```python
from build123d import *

# Parameters (mm, degrees)
SKETCH1_W             = 32
SKETCH1_H             = 48
BOSS_EXTRUDE1_DEPTH   = 26
SHELL1_T              = -2
SKETCH2_W             = 26.2
SKETCH2_H             = 24
CUT_EXTRUDE1_DEPTH    = 20
CHAMFER1_SIZE         = 2.5
CHAMFER1_SIZE2        = 2.979383981
CHAMFER1_PART_2_SIZE  = 2.5
CHAMFER1_PART_2_SIZE2 = 2.979383981
CHAMFER3_SIZE         = 2.5
SKETCH5_W             = 27
SKETCH5_H             = 2.432389293
BOSS_EXTRUDE3_DEPTH   = 10
CHAMFER4_SIZE         = 5
SKETCH6_R             = 8.805
CUT_EXTRUDE3_DEPTH    = 10


with BuildPart() as part:
    # Sketch1 → Boss-Extrude1 (new body)
    with BuildSketch(Plane(origin=(0, 0, 0), x_dir=(1, 0, 0), z_dir=(0, 1, 0))):
        Rectangle(SKETCH1_W, SKETCH1_H)
    extrude(amount=BOSS_EXTRUDE1_DEPTH)

    # Shell1
    shell1_openings = [part.faces().sort_by_distance(p)[0] for p in [
        (0, 26, 0),
    ]]
    offset(amount=SHELL1_T, openings=shell1_openings, kind=Kind.INTERSECTION)

    # Sketch2 → Cut-Extrude1 (cut)
    with BuildSketch(Plane(origin=(0, 0, -24), x_dir=(-1, 0, 0), z_dir=(0, 0, -1))):
        with Locations((0, 14)):
            Rectangle(SKETCH2_W, SKETCH2_H)
    extrude(amount=-CUT_EXTRUDE1_DEPTH, mode=Mode.SUBTRACT)

    # Chamfer1
    chamfer1_edges = [part.edges().sort_by_distance(p)[0] for p in [
        (16, 13, 24),
    ]]
    chamfer1_side = [part.faces().sort_by_distance(p)[0] for p in [
        (0, 13, 24),
    ]]
    chamfer(chamfer1_edges, length=CHAMFER1_SIZE, length2=CHAMFER1_SIZE2, reference=chamfer1_side[0])

    # Chamfer1 part 2
    chamfer1_part_2_edges = [part.edges().sort_by_distance(p)[0] for p in [
        (-16, 13, 24),
    ]]
    chamfer1_part_2_side = [part.faces().sort_by_distance(p)[0] for p in [
        (-16, 13, 0),
    ]]
    chamfer(chamfer1_part_2_edges, length=CHAMFER1_PART_2_SIZE, length2=CHAMFER1_PART_2_SIZE2, reference=chamfer1_part_2_side[0])

    # Chamfer3
    chamfer3_edges = [part.edges().sort_by_distance(p)[0] for p in [
        (-16, 13, -24),
        (16, 13, -24),
    ]]
    chamfer(chamfer3_edges, length=CHAMFER3_SIZE)

    # Sketch5 → Boss-Extrude3 (add)
    with BuildSketch(Plane(origin=(0, 0, -24), x_dir=(-1, 0, 0), z_dir=(0, 0, -1))):
        with Locations((0, 1.216194646)):
            Rectangle(SKETCH5_W, SKETCH5_H)
    extrude(amount=BOSS_EXTRUDE3_DEPTH)

    # Chamfer4
    chamfer4_edges = [part.edges().sort_by_distance(p)[0] for p in [
        (13.5, 1.216194647, -34),
        (-13.5, 1.216194647, -34),
    ]]
    chamfer(chamfer4_edges, length=CHAMFER4_SIZE)

    # Sketch6 → Cut-Extrude3 (cut)
    with BuildSketch(Plane.XY.offset(24)):
        with Locations((0, 16.205)):
            Circle(SKETCH6_R)
    extrude(amount=-CUT_EXTRUDE3_DEPTH, mode=Mode.SUBTRACT)


solid = part.part
```
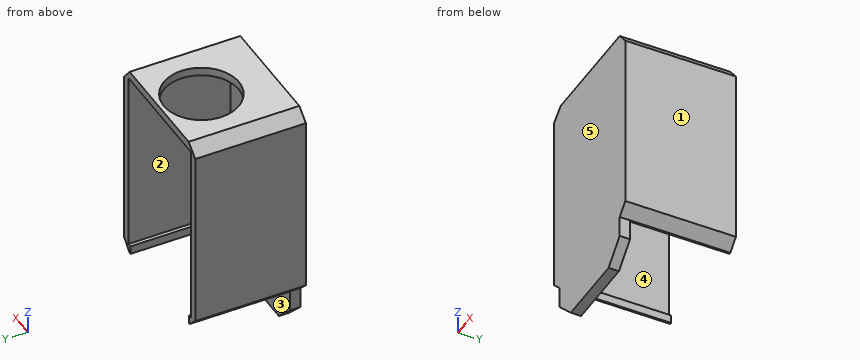
The listing builds one solid part. Answer for the finished solid, in the listing's coordinates (mm). Face numbers are marked on the shaded views. A direction names the side the tool comes from. Coordinates: 2 decimals unless noted, no trailing zeros. Write each loop counter-clockwise with the first axis right and the second up, starting at its lowest first coordinate (ties: lowest second). Pieces come first, ordered by that corner, then holes.
Q1. Section C-C, the plane y = 14.75 is taken. Write down the section's boundary in (x, z), then the cut area to 3 significant figures.
Returned:
outline: (-16, -21.5) - (-13.5, -24) - (-13.1, -24) - (-13.1, -22) - (-14, -22) - (-14, 22) - (-8.68, 22) - (-8.68, 24) - (-13.02, 24) - (-16, 21.5) - close; (8.68, 22) - (14, 22) - (14, -22) - (13.1, -22) - (13.1, -24) - (13.5, -24) - (16, -21.5) - (16, 21.02) - (13.5, 24) - (8.68, 24) - close
area: 203 mm2
Q2. Which of the six approach directions +Z, -Z, +X, -X, +Y, -Y give full straight-line access (tool end or side, diameter ignored) to the marked faces 4 and 5?
Returned:
face 4: +Y
face 5: +Z, -Z, +X, -X, -Y
Q3. Find the intervals of material crossed by line 1 along X through (y, z) = (20, -1.5); line 2 along Y through (x, z) = (0, 22.55); line 3 along Z through (x, y) = (3, 2.25), in increasing order.
Returned:
line 1: x = -16 to -14, 14 to 16
line 2: y = 0 to 7.4, 25.01 to 26
line 3: z = -34 to -24, 22 to 24
Q4. Section B-B, the plane z = -9 is taken. Write down the section's boundary in (x, y), then the cut area to 3 significant figures.
Returned:
outline: (-16, 0) - (16, 0) - (16, 26) - (14, 26) - (14, 2) - (-14, 2) - (-14, 26) - (-16, 26) - close
area: 160 mm2
Q5. Section A-A, the plane x = 9.5 is taken. Write down the section's boundary in (y, z).
Returned:
outline: (0, -33) - (2.43, -33) - (2.43, -24) - (2, -24) - (2, 22) - (26, 22) - (26, 24) - (0, 24) - close
Q6. Section D-D, the plane x = 0 is taken. Write down the section's boundary in (y, z), then the cut area to 3 significant figures.
Returned:
outline: (0, -34) - (2.43, -34) - (2.43, -24) - (2, -24) - (2, 22) - (7.4, 22) - (7.4, 24) - (0, 24) - close; (25.01, 22) - (26, 22) - (26, 24) - (25.01, 24) - close
area: 133 mm2
Q7. The mould has two halves that part along X. Classify the marked faces 1, 2 and 3: released by +X, released by -X, zero draft, split by the parting line, or undercut.
Returned:
face 1: released by +X
face 2: undercut
face 3: zero draft
Q8. Given P1, Ø0.5, axis at x = -13.5, y = 10.5, coming from the +Z side; P2, Ø5, axis at x = 3, z = -27, coming from the +Y side; P3, Ø1, axis at x = -8, z = 4, coming from the +Y side, each flat-ended and moving along its own axis, determine where each tip first touches the part or whether it passes through.
Returned:
P1: stops at z = 23.81
P2: stops at y = 2.43
P3: stops at y = 2
